```python
from build123d import *

# Parameters (mm, degrees)
EXTRUDE_THIN2_DEPTH = 1028.7


with BuildPart() as part:
    # Sketch1 → Extrude-Thin2 (new body)
    with BuildSketch(Plane(origin=(0, 0, 0), x_dir=(0, 0, -1), z_dir=(1, 0, 0))):
        with BuildLine():
            Line((22.252869444, 65.934166667), (-9.497130556, 65.934166667))
            ThreePointArc((-9.497130556, 65.934166667), (-11.742194586, 65.004230697), (-12.672130556, 62.759166667))
            Line((-12.672130556, 62.759166667), (-12.672130556, -7.090833333))
            ThreePointArc((-12.672130556, -7.090833333), (-11.742194586, -9.335897364), (-9.497130556, -10.265833333))
            Line((-9.497130556, -10.265833333), (22.252869444, -10.265833333))
            ThreePointArc((22.252869444, -10.265833333), (24.497933475, -9.335897364), (25.427869444, -7.090833333))
            Line((25.427869444, -7.090833333), (25.427869444, 62.759166667))
            ThreePointArc((25.427869444, 62.759166667), (24.497933475, 65.004230697), (22.252869444, 65.934166667))
        make_face()
        with BuildLine():
            Line((22.252869444, 64.283166667), (-9.497130556, 64.283166667))
            ThreePointArc((-9.497130556, 64.283166667), (-10.57476129, 63.836797401), (-11.021130556, 62.759166667))
            Line((-11.021130556, 62.759166667), (-11.021130556, -7.090833333))
            ThreePointArc((-11.021130556, -7.090833333), (-10.57476129, -8.168464068), (-9.497130556, -8.614833333))
            Line((-9.497130556, -8.614833333), (22.252869444, -8.614833333))
            ThreePointArc((22.252869444, -8.614833333), (23.330500179, -8.168464068), (23.776869444, -7.090833333))
            Line((23.776869444, -7.090833333), (23.776869444, 62.759166667))
            ThreePointArc((23.776869444, 62.759166667), (23.330500179, 63.836797401), (22.252869444, 64.283166667))
        make_face(mode=Mode.SUBTRACT)
    extrude(amount=EXTRUDE_THIN2_DEPTH)


solid = part.part
```
Check sheet for the modelled part. Datum: model origin and axes. Units: mm. A direction names the side the tool comes from. Round coordinates to 2 decimals unless told otherwise and drop trailing zeros. Loops run counter-clockwise (first coordinate to the right, second up) from the corner with the lowest first, then second, coordinate; pieces in that order, holes last. Notation, with made-up numbers: (-19, -1.75) - (37, -1.75) arc R38 ccw to (37, 36.25) - close; hole circle Ø3 at (-4.75, -17.5). An arc over 180 degrees is marked (long way). Answer as a JSON object with one key per item and string values. Group by question number.
Q1. Scan lines: line 1 along Z through (x, y) = (690.5, 14.5); line 2 along Y through (x, z) = (263.5, -16). Record each from-to range of solid material in increasing order. Write a range as [from, to].
Q2. Sectioned sample at A-A, the plane y = 52. Enter the section's corners in (x, z).
Q3. Sectioned sample at C-C, the plane x = 153.5. Enter the section's corners in (y, z) (3 decimals).
Q4. Set-up check for faces 5 (the face through (507, -8.615, -6)), 6 (the face through (0, 28, 12)): record each of +Z, -Z, +X, -X, +Y, -Y from which the full face is reachable in a straight line by a thin tool's end or side.
Q5. Gauge pin test, flat end, axial feed: P1, Ø12, axis at y = 36, z = 6, coming from the -X side. Record the tip position at first contact, or that the pin passes through.
Q6. Sectioned sample at B-B, the plane z = -12.5. Enter the section's corners in (x, y), plus the area to 3 significant figures.
Q7. Mould release check, pull along Y, two halves, no side actions. Record for faces 1 (the face through (507, 27, -25.428)), 2 (the face through (507, 28, 11.021)), 3 (the face through (507, 27, -23.777)), 4 (the face through (507, -10.266, -6)): released by +Y, released by -Y, zero draft, split by the parting line, or undercut.
Solution:
{
 "1": {"line 1": "z = [-25.43, -23.78], [11.02, 12.67]", "line 2": "y = [-10.27, -8.61], [64.28, 65.93]"},
 "2": {"outline": "(0, -25.43) - (1028.7, -25.43) - (1028.7, -23.78) - (0, -23.78) - close; (0, 11.02) - (1028.7, 11.02) - (1028.7, 12.67) - (0, 12.67) - close"},
 "3": {"outline": "(-10.266, -22.253) arc R3.175 ccw to (-7.091, -25.428) - (62.759, -25.428) arc R3.175 ccw to (65.934, -22.253) - (65.934, 9.497) arc R3.175 ccw to (62.759, 12.672) - (-7.091, 12.672) arc R3.175 ccw to (-10.266, 9.497) - close; hole (-8.615, -22.253) arc R1.524 ccw to (-7.091, -23.777) - (62.759, -23.777) arc R1.524 ccw to (64.283, -22.253) - (64.283, 9.497) arc R1.524 ccw to (62.759, 11.021) - (-7.091, 11.021) arc R1.524 ccw to (-8.615, 9.497) - close"},
 "4": {"face 5": "+X, -X", "face 6": "+Z, -Z, -X, +Y, -Y"},
 "5": {"P1": "stops at x = 0"},
 "6": {"outline": "(0, -10.27) - (1028.7, -10.27) - (1028.7, -8.61) - (0, -8.61) - close; (0, 64.28) - (1028.7, 64.28) - (1028.7, 65.93) - (0, 65.93) - close", "area": "3,400 mm²"},
 "7": {"face 1": "zero draft", "face 2": "undercut", "face 3": "undercut", "face 4": "released by -Y"}
}
